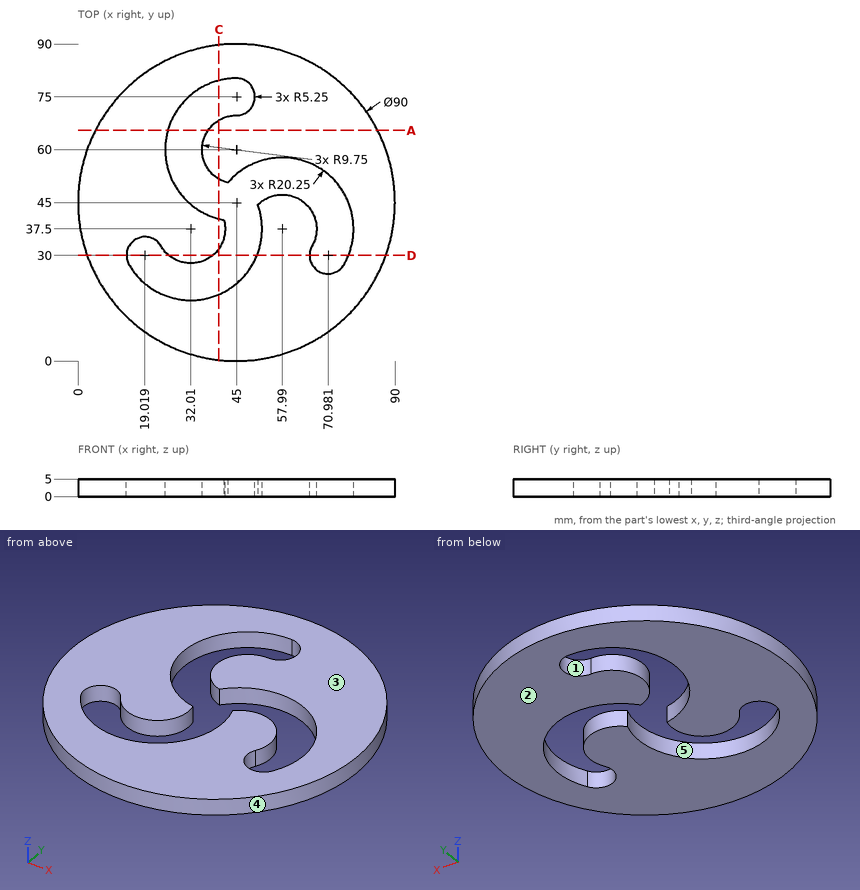
Input: dimensioned drawing with shaded views. Units: mm. Origin: part minimum x, y, z. A direction names the side the tool comes from. Round coordinates to 2 decimals unless told otherwise and drop trailing zeros. Loops run counter-clockwise (first coordinate to the right, second up) from the corner with the lowest first, then second, coordinate; pieces in that order, holes last. Notation, with made-up numbers: (66, 70.25) -> (78, 70.25) arc R29 cw to (78, 97.25) -> close; hole circle Ø8 at (66, 0). An arc over 180 degrees is marked (long way). Use one line per item in the form item = value. Start each with the question number.
1) Draft query along X for the marked faces 3, 4 and 5. Return one class per face: released by +X, released by -X, zero draft, split by the parting line, or undercut.
2) First-contact query: P1, Ø1, axis at x = 18, z = 1.5, coming from the +Y side; P2, Ø2, axis at y = 36, z = 4, coming from the +X side. Flat tips, straight axial feed; report the tip coordinate or a pass-through.
3) Access query for the marked faces 1 and 2. Directions: +Z, -Z, +X, -X, +Y, -Y. A direction counts if a zero-diameter tool reaches every point of the face in a straight line with its end or side. Return the directions, or none.
4) Section D-D on y = 30. Output: boundary loops of the cut face in (x, z), then the cut area to 3 significant figures.
5) Line query: L1, parallel to X at y = 52.5, z = 1.7 (1 decimal); L2, parallel to X at y = 46, z = 0.9 (1 decimal); L3, parallel to Y at x = 33.5, z = 1.6 (1 decimal). Output: solid intervals per line, ascending.
6) Section A-A on y = 65.5. Output: boundary loops of the cut face in (x, z).
7) Section C-C on x = 40. Output: boundary loops of the cut face in (y, z).
Response:
q1.face_3 = zero draft
q1.face_4 = split by the parting line
q1.face_5 = undercut
q2.P1 = 81.37
q2.P2 = 89.28
q3.face_1 = +Z, -Z
q3.face_2 = -Z, +X, -X, +Y, -Y
q4.outline = (2.57, 0) -> (13.77, 0) -> (13.77, 5) -> (2.57, 5) -> close; (25.78, 0) -> (38.24, 0) -> (38.24, 5) -> (25.78, 5) -> close; (50.82, 0) -> (65.73, 0) -> (65.73, 5) -> (50.82, 5) -> close; (76.8, 0) -> (87.43, 0) -> (87.43, 5) -> (76.8, 5) -> close
q4.area = 246 mm^2
q5.L1 = 0.6 to 26.2, 38.8 to 44.4, 71.6 to 89.4
q5.L2 = 0 to 30.4, 53.2 to 62.8, 76.4 to 90
q5.L3 = 1.5 to 17.3, 27.9 to 43.3, 76.7 to 88.5
q6.outline = (4.94, 0) -> (25.51, 0) -> (25.51, 5) -> (4.94, 5) -> close; (36.95, 0) -> (85.06, 0) -> (85.06, 5) -> (36.95, 5) -> close
q7.outline = (0.28, 0) -> (18.89, 0) -> (18.89, 5) -> (0.28, 5) -> close; (31.91, 0) -> (40.38, 0) -> (40.38, 5) -> (31.91, 5) -> close; (51.63, 0) -> (68.37, 0) -> (68.37, 5) -> (51.63, 5) -> close; (79.62, 0) -> (89.72, 0) -> (89.72, 5) -> (79.62, 5) -> close
